Autodesk Inventor part; units mm, degrees
ref_plane "YZ Plane" through (0, 0, 0) normal (1, 0, 0) x (0, 1, 0)
ref_plane "XZ Plane" through (0, 0, 0) normal (0, 1, 0) x (-1, 0, 0)
ref_plane "XY Plane" through (0, 0, 0) normal (0, 0, 1) x (1, 0, 0)
sketch "スケッチ1" plane through (0, 0, 0) normal (0, 1, 0) x (-1, 0, 0)
  line L0 (0, 0) -> (72, 0)
  line L1 (72, 0) -> (72, -47)
  line L2 (72, -47) -> (0, -47)
  line L3 (0, -47) -> (0, 0)
  dimension "d0" = 72
  dimension "d1" = 47
extrude "押し出し1" add sketch "スケッチ1" along normal blind 3
sketch "スケッチ2" plane through (0, 3, 0) normal (0, 1, 0) x (1, 0, 0)
  line L0 (-72, 47) -> (-72, 0)
  line L1 (0, 47) -> (-72, 47)
  line L2 (-72, 0) -> (0, 0)
  line L3 (0, 0) -> (0, 47)
  point P0 (-69, 3)
  point P1 (-69, 44)
  point P2 (-3, 3)
  point P3 (-3, 44)
  dimension "d4" = 3
  dimension "d5" = 3
  dimension "d6" = 3
  dimension "d7" = 3
  dimension "d15" = 41
  dimension "d16" = 66
hole "穴1" at (-69, 3, -3) at (-69, 3, -44) at (-3, 3, -3) at (-3, 3, -44) direction (0, -1, 0) diameter 3.2 depth 3
properties part number "mainBoard" material "エポキシ樹脂"
Build history of the part. All positions in model axes, mm. Coordinates: 2 decimals unless noted, no trailing zeros. Write each loop counter-clockwise with the first axis right and the second up, starting at its lowest first coordinate (ties: lowest second). Pieces come first, ordered by that corner, then holes.
(1) Cut at B-B on x = -3. List the corners of the cut face in (y, z).
(2) Cut at A-A on z = -44. List the corners of the cut face in (x, y).
(3) Drill centre lines: line 1 (X direction, y = 1.15, z = -44); line 2 (Z direction, x = -69, y = 2.1); line 3 (X direction, y = 2.5, z = -45). Where is each one in solid material? Low to high.
(4) Mould opens along Z. For faces 1 (the flat face through (-35, 0, -23)), 2 (the cylindrical face through (-1.44, 1.48, -3.35)), 3 (the flat face through (-35, 1, 0)) say: pulls with the +Z half, pulls with the -Z half, needs draft (parallel to the pull), parting line crosses it, or undercut.
Working result:
1. outline: (0, -47) - (3, -47) - (3, -45.6) - (0, -45.6) - close; (0, -42.4) - (3, -42.4) - (3, -4.6) - (0, -4.6) - close; (0, -1.4) - (3, -1.4) - (3, 0) - (0, 0) - close
2. outline: (-72, 0) - (-70.6, 0) - (-70.6, 3) - (-72, 3) - close; (-67.4, 0) - (-4.6, 0) - (-4.6, 3) - (-67.4, 3) - close; (-1.4, 0) - (0, 0) - (0, 3) - (-1.4, 3) - close
3. line 1: x = -72 to -70.6, -67.4 to -4.6, -1.4 to 0
3. line 2: z = -47 to -45.6, -42.4 to -4.6, -1.4 to 0
3. line 3: x = -72 to -70.25, -67.75 to -4.25, -1.75 to 0
4. face 1: needs draft
4. face 2: undercut
4. face 3: pulls with the +Z half
